Geometry check sheet. Reference: the model listing, model coordinates, mm. Face numbers are marked on the shaded views. Coordinates: 2 decimals unless noted, no trailing zeros. Write each loop counter-clockwise with the first axis right and the second up, starting at its lowest first coordinate (ties: lowest second). Pieces come first, ordered by that corner, then holes. Notation, with made-up numbers: M 50,18 L 61,18 A18 cw 61,38 Z; hole C 4,-21.5 d1. An arc over 180 degrees is marked long. Write each question's results on one line, items separated by ' | '.
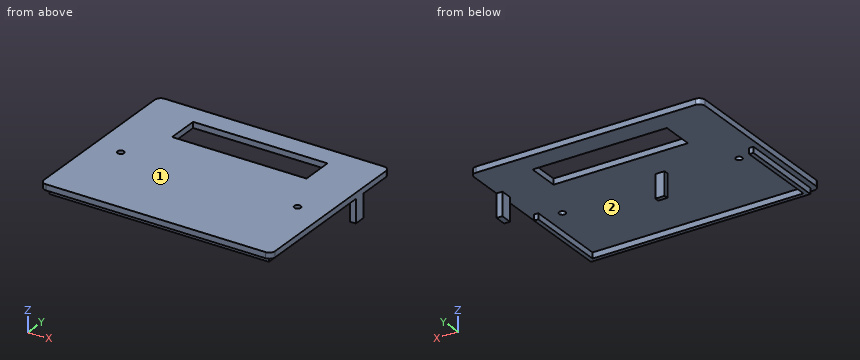
```python
from build123d import *

# Parameters (mm, degrees)
F1_DEPTH = 2
F0_R     = 3
F0_R_2   = 1.1
F2_DEPTH = 2
F0_W     = 3.1642657705
F0_H     = 1.4890261218
F3_DEPTH = 10
F4_DEPTH = 4
F5_R     = 2


with BuildPart() as f1:
    # F0 (on Top) → F1 (new body)
    with BuildSketch(Plane.XY):
        Polygon((-37.55, -13.0740804598), (-37.55, -12.1), (-37.55, 13.5259195402), (37.55, 13.5259195402), (37.55, 2.0000108369), (39.55, 2.0000108369), (39.55, 15.7519578086), (-39.5226512551, 15.7519578086), (-39.5226512551, -46.2480421914), (39.55, -46.2480421914), (39.55, -1.9999891631), (37.55, -1.9999891631), (37.55, -13.0740804598), (-4.9305087887, -13.0740804598), (-4.9305087887, -14.5631065816), (36.1, -14.5631065816), (37.55, -14.5631065816), (37.55, -44.3981406778), (-37.55, -44.3981406778), (-37.55, -14.5631065816), (-36.1, -14.5631065816), (-8.0947745591, -14.5631065816), (-8.0947745591, -13.0740804598), align=None)
    extrude(amount=-F1_DEPTH)

    # F0 (on Top) → F2 (join)
    with BuildSketch(Plane.XY):
        Polygon((-4.9305087887, -14.5631065816), (-8.0947745591, -14.5631065816), (-36.1, -14.5631065816), (-36.1, -42.9981406778), (36.1, -42.9981406778), (36.1, -14.5631065816), align=None)
        with Locations((-30.2370786667, -18.2506926358)):
            Circle(F0_R, mode=Mode.SUBTRACT)
        with Locations((30.2370786667, -18.2506926358)):
            Circle(F0_R, mode=Mode.SUBTRACT)
        Polygon((-37.55, 13.5259195402), (-37.55, -12.1), (-37.55, -13.0740804598), (-8.0947745591, -13.0740804598), (-4.9305087887, -13.0740804598), (37.55, -13.0740804598), (37.55, -1.9999891631), (37.55, 2.0000108369), (37.55, 13.5259195402), align=None)
        Polygon((36.1, 12.1), (36.1, -12.1), (-36.1, -12.1), (-36.1, 12.1), (-25.6, 12.1), (29.1, 12.1), align=None, mode=Mode.SUBTRACT)
        Polygon((-36.1, -12.1), (36.1, -12.1), (36.1, 12.1), (29.1, 12.1), (-25.6, 12.1), (-36.1, 12.1), align=None)
        with BuildLine():
            ThreePointArc((-23, 0.1033370453), (-28.1971127107, 0.0983324043), (-25.6, 4.6))
            ThreePointArc((-25.6, 4.6), (-24.0983324043, 4.1971127107), (-23, 3.0966629547))
            Line((-23, 3.0966629547), (-23, 8.5))
            Line((-23, 8.5), (0, 8.5))
            Line((0, 8.5), (23, 8.5))
            Line((23, 8.5), (23, -2.5))
            Line((23, -2.5), (-23, -2.5))
            Line((-23, -2.5), (-23, 0.1033370453))
        make_face(mode=Mode.SUBTRACT)
        with BuildLine():
            ThreePointArc((32.1000297599, 2.1), (26.978658613, -0.021341387), (29.1, 5.1000297599))
            ThreePointArc((29.1, 5.1000297599), (31.221341387, 4.221341387), (32.1000297599, 2.1))
        make_face(mode=Mode.SUBTRACT)
        Polygon((-36.1, -42.9981406778), (-36.1, -14.5631065816), (-37.55, -14.5631065816), (-37.55, -44.3981406778), (37.55, -44.3981406778), (37.55, -14.5631065816), (36.1, -14.5631065816), (36.1, -42.9981406778), align=None)
        with BuildLine():
            ThreePointArc((32.1000297599, 2.1), (31.221341387, 4.221341387), (29.1, 5.1000297599))
            ThreePointArc((29.1, 5.1000297599), (26.978658613, -0.021341387), (32.1000297599, 2.1))
        make_face()
        with BuildLine():
            ThreePointArc((30.2, 2.1), (28.3221825407, 1.3221825407), (29.1, 3.2))
            ThreePointArc((29.1, 3.2), (29.8778174593, 2.8778174593), (30.2, 2.1))
        make_face(mode=Mode.SUBTRACT)
        with Locations((30.2370786667, -18.2506926358)):
            Circle(F0_R)
        with Locations((30.2370786667, -18.2506926358)):
            Circle(F0_R_2, mode=Mode.SUBTRACT)
        with Locations((-30.2370786667, -18.2506926358)):
            Circle(F0_R)
        with Locations((-30.2370786667, -18.2506926358)):
            Circle(F0_R_2, mode=Mode.SUBTRACT)
        with BuildLine():
            Line((-25.6, 2.7), (-25.6, 4.6))
            ThreePointArc((-25.6, 4.6), (-28.1971127107, 0.0983324043), (-23, 0.1033370453))
            Line((-23, 0.1033370453), (-23, 1.6))
            Line((-23, 1.6), (-24.5, 1.6))
            ThreePointArc((-24.5, 1.6), (-26.3778174593, 0.8221825407), (-25.6, 2.7))
        make_face()
        with BuildLine():
            ThreePointArc((-23, 3.0966629547), (-24.0983324043, 4.1971127107), (-25.6, 4.6))
            Line((-25.6, 4.6), (-25.6, 2.7))
            ThreePointArc((-25.6, 2.7), (-24.8221825407, 2.3778174593), (-24.5, 1.6))
            Line((-24.5, 1.6), (-23, 1.6))
            Line((-23, 1.6), (-23, 3.0966629547))
        make_face()
        with BuildLine():
            ThreePointArc((30.2, 2.1), (29.8778174593, 2.8778174593), (29.1, 3.2))
            ThreePointArc((29.1, 3.2), (28.3221825407, 1.3221825407), (30.2, 2.1))
        make_face()
        with BuildLine():
            Line((-25.6, 1.6), (-25.6, 2.7))
            ThreePointArc((-25.6, 2.7), (-26.3778174593, 0.8221825407), (-24.5, 1.6))
            Line((-24.5, 1.6), (-25.6, 1.6))
        make_face()
        with BuildLine():
            ThreePointArc((-24.5, 1.6), (-24.8221825407, 2.3778174593), (-25.6, 2.7))
            Line((-25.6, 2.7), (-25.6, 1.6))
            Line((-25.6, 1.6), (-24.5, 1.6))
        make_face()
    extrude(amount=-F2_DEPTH)

    # F0 (on Top) → F3 (join)
    with BuildSketch(Plane.XY):
        Polygon((39.55, 2.0000108369), (37.55, 2.0000108369), (37.55, -1.9999891631), (39.55, -1.9999891631), (39.55, 1.08369e-05), align=None)
        with Locations((-6.5126416739, -13.8185935207)):
            Rectangle(F0_W, F0_H)
    extrude(amount=-F3_DEPTH)

    # F0 (on Top) → F4 (join)
    with BuildSketch(Plane.XY):
        Polygon((-36.1, -42.9981406778), (-36.1, -14.5631065816), (-37.55, -14.5631065816), (-37.55, -44.3981406778), (37.55, -44.3981406778), (37.55, -14.5631065816), (36.1, -14.5631065816), (36.1, -42.9981406778), align=None)
    extrude(amount=-F4_DEPTH)

    # F5
    f5_edges = [f1.edges().sort_by_distance(p)[0] for p in [
        (-39.522651, 15.751958, -1),
        (39.55, 15.751958, -1),
        (39.55, -46.248042, -1),
        (-39.522651, -46.248042, -1),
    ]]
    fillet(f5_edges, radius=F5_R)


solid = f1.part
```
Q1. Scan lines: probe 1 along X at (y, z) = (-28, -3.75); probe 2 along Z at (x, y) = (26, 2); probe 3 along Y at (x, z) = (-29.5, -0.75). Record each from-to range of solid material in increasing order.
Geometry check:
probe 1: x = -37.55 to -36.1, 36.1 to 37.55 | probe 2: z = -2 to 0 | probe 3: y = -46.25 to -19.07, -17.43 to 15.75
Q2. Sectioned sample at C-C on x = 18. Record the cut outline in (y, z), and give its area (3 significant figures).
Geometry check:
outline: M -46.25,-2 L -44.4,-2 L -44.4,-4 L -43,-4 L -43,-2 L -2.5,-2 L -2.5,0 L -46.25,0 Z; M 8.5,-2 L 15.75,-2 L 15.75,0 L 8.5,0 Z | area: 105 mm2
Q3. Sectioned sample at B-B on z = -5.25. Record the cut outline in (x, y).
Geometry check:
outline: M -8.09,-14.56 L -4.93,-14.56 L -4.93,-13.07 L -8.09,-13.07 Z; M 37.55,-2 L 39.55,-2 L 39.55,2 L 37.55,2 Z
Q4. Depth check by flat-ended pin: P1, Ø2.5, axis at x = -30.24, y = -18.25, coming from the -Z side; P2, Ø3.5, axis at x = -6, z = -6.5, coming from the -Y side; P3, Ø5, axis at y = -35, z = -5, coming from the -X side. Enter the tip coordinate at first touch or a pass-through.
Geometry check:
P1: stops at z = -2 | P2: stops at y = -14.56 | P3: stops at x = -37.55
Q5. Sectioned sample at A-A on y = 6. Record the cut outline in (x, z), and give its area (3 significant figures).
Geometry check:
outline: M -39.52,-2 L -23,-2 L -23,0 L -39.52,0 Z; M 23,-2 L 39.55,-2 L 39.55,0 L 23,0 Z | area: 66.1 mm2
Q6. Mould release check, pull along X, two halves, no side actions. Record for the marked faces 1 and 2: pulls with the +X half, pulls with the -X half, needs draft (parallel to the pull), parting line crosses it, or undercut.
Geometry check:
face 1: needs draft | face 2: undercut
Q7. Sectioned sample at D-D on y = -40.5. Record the cut outline in (x, z), and give its area (3 significant figures).
Geometry check:
outline: M -39.52,-2 L -37.55,-2 L -37.55,-4 L -36.1,-4 L -36.1,-2 L 36.1,-2 L 36.1,-4 L 37.55,-4 L 37.55,-2 L 39.55,-2 L 39.55,0 L -39.52,0 Z | area: 164 mm2
